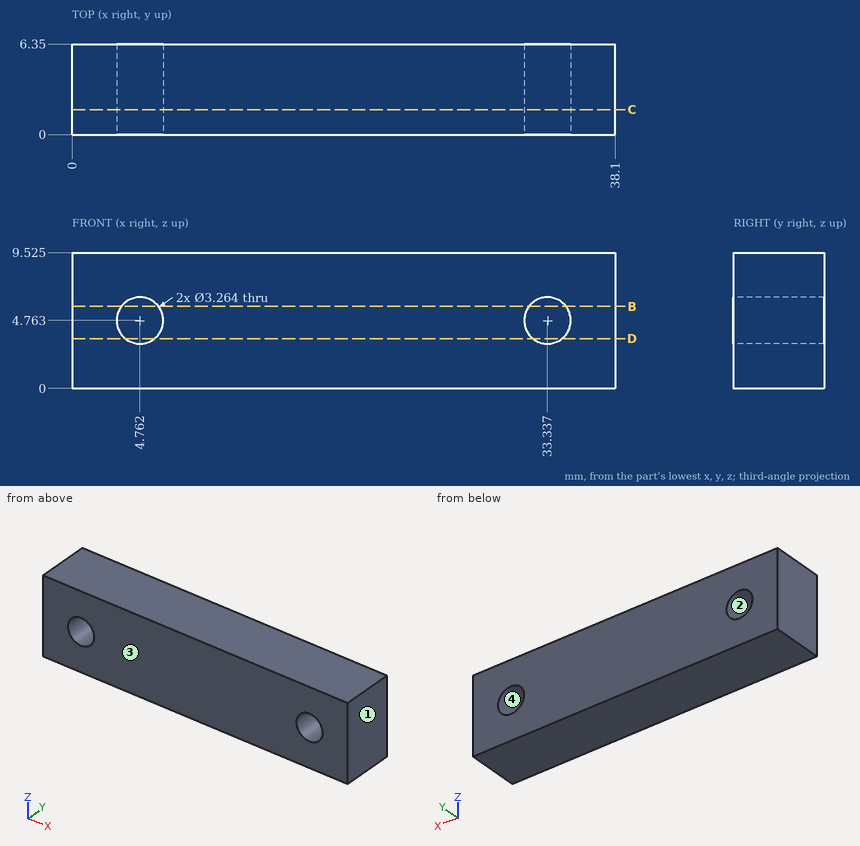
Input: dimensioned drawing with shaded views. Units: mm. Origin: part minimum x, y, z. Give positions to 0.01 mm unless a question says otherwise; leave off trailing zeros. Order: outer loops, then holes, each group sorted by start corner. A loop starts at its lowest first (then second) coordinate and runs counter-clockwise, first axis right, second up. Notation, with made-up numbers: (-15.75, 0) -> (38.25, 0) arc R15 ccw to (38.25, 4) -> close; hole circle Ø7 at (84, -13). An arc over 180 degrees is marked (long way). Use a Markdown table: item, result.
1) Mould query, pull axis X, two halves, no side actions, for the marked faces 1, 2, 3 and 4. Classes: +X half, -X half, draft (parallel to the pull), parting line (faces both ways), or undercut.
Answer list:
| item | result |
|---|---|
| face 1 | +X half |
| face 2 | undercut |
| face 3 | draft |
| face 4 | undercut |
2) Ray query, line 1 along X through (y, z) = (2.75, 3.75) (1 decimal); line 2 along X through (y, z) = (5.5, 4) (1 decimal); line 3 along Z through (x, y) = (34.5, 1.75) (1 decimal). Return the intervals inside material, ascending. Write a range as [from, to].
Answer list:
| item | result |
|---|---|
| line 1 | [0, 3.5], [6, 32.1], [34.6, 38.1] |
| line 2 | [0, 3.3], [6.2, 31.9], [34.8, 38.1] |
| line 3 | [0, 3.6], [5.9, 9.5] |
3) Contact query for a flat-ended pin moving along its axis: P1, Ø2, axis at x = 4.76, z = 4.76, coming from the +Y side. Output: stop coordinate, or through.
Answer list:
| item | result |
|---|---|
| P1 | through |
4) Section query C-C, the plane y = 1.75. Return the cut outline in (x, z) (1 decimal).
Answer list:
| item | result |
|---|---|
| outline | (0, 0) -> (38.1, 0) -> (38.1, 9.5) -> (0, 9.5) -> close; hole circle Ø3.3 at (4.8, 4.8); hole circle Ø3.3 at (33.3, 4.8) |
5) Section query D-D, the plane z = 3.5. Return the cut outline in (x, y), then the cut area to 3 significant figures.
Answer list:
| item | result |
|---|---|
| outline | (0, 0) -> (3.73, 0) -> (3.73, 6.35) -> (0, 6.35) -> close; (5.8, 0) -> (32.3, 0) -> (32.3, 6.35) -> (5.8, 6.35) -> close; (34.37, 0) -> (38.1, 0) -> (38.1, 6.35) -> (34.37, 6.35) -> close |
| area | 216 mm² |
6) Section query B-B, the plane z = 5.75. Return the cut outline in (x, y), then the cut area to 3 significant figures.
Answer list:
| item | result |
|---|---|
| outline | (0, 0) -> (3.46, 0) -> (3.46, 6.35) -> (0, 6.35) -> close; (6.06, 0) -> (32.04, 0) -> (32.04, 6.35) -> (6.06, 6.35) -> close; (34.64, 0) -> (38.1, 0) -> (38.1, 6.35) -> (34.64, 6.35) -> close |
| area | 209 mm² |
